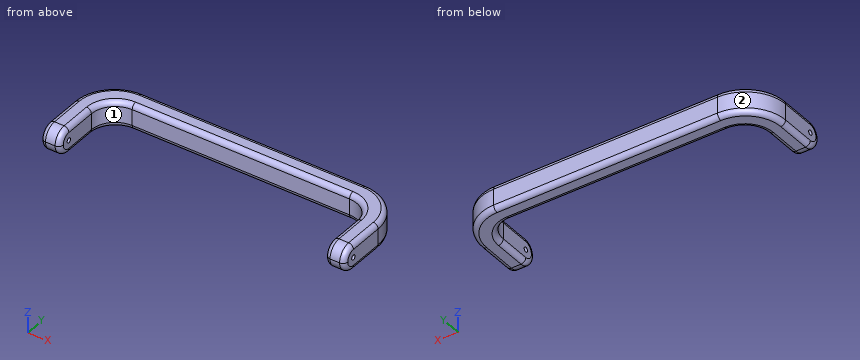
```python
from build123d import *

# Parameters (mm, degrees)
F1_DEPTH = 16
F2_R     = 15
F3_R     = 25
F4_R     = 7.99999
F5_R     = 1.5
F6_DEPTH = 250
F7_R     = 3


# Not quite as in the source:
# - a fillet or chamfer is up to 0.001 mm smaller than in the source, because OpenCascade refuses the exact size


with BuildPart() as f1:
    # F0 (on Top) → F1 (new body)
    with BuildSketch(Plane.XY):
        Polygon((95, 35.7796452148), (0, 35.7796452148), (-95, 35.7796452148), (-95, -19.2203547852), (-83, -19.2203547852), (-83, 23.7796452148), (0, 23.7796452148), (83, 23.7796452148), (83, -19.2203547852), (95, -19.2203547852), align=None)
    extrude(amount=F1_DEPTH)

    # F2
    f2_edges = [f1.edges().sort_by_distance(p)[0] for p in [
        (-83, 23.779645, 8),
        (83, 23.779645, 8),
    ]]
    fillet(f2_edges, radius=F2_R)

    # F3
    f3_edges = [f1.edges().sort_by_distance(p)[0] for p in [
        (-95, 35.779645, 8),
        (95, 35.779645, 8),
    ]]
    fillet(f3_edges, radius=F3_R)

    # F4 (radius 8 in the source; OpenCascade refuses exactly that, so slightly less here)
    f4_edges = [f1.edges().sort_by_distance(p)[0] for p in [
        (-89, -19.220355, 16),
        (-89, -19.220355, 0),
        (89, -19.220355, 16),
        (89, -19.220355, 0),
    ]]
    fillet(f4_edges, radius=F4_R)

    # F5 (on face) → F6 (cut)
    with BuildSketch(Plane.YZ.offset(95)):
        with Locations((-11.2203547852, 8)):
            Circle(F5_R)
    extrude(amount=-F6_DEPTH, mode=Mode.SUBTRACT)

    # F7
    f7_edges = [f1.edges().sort_by_distance(p)[0] for p in [
        (-95, -0.22036, 0),
        (-89, -11.220365, 0),
        (-87.67767, 28.457315, 0),
        (-83, -1.22036, 0),
        (0, 35.779645, 0),
        (-78.606602, 19.386247, 0),
        (87.67767, 28.457315, 0),
        (0, 23.779645, 0),
        (95, -0.22036, 0),
        (78.606602, 19.386247, 0),
        (89, -11.220365, 0),
        (83, -1.22036, 0),
    ]]
    fillet(f7_edges, radius=F7_R)


solid = f1.part
```
The listing builds one solid part. Answer for the finished solid, in the listing's coordinates (mm). Face numbers are marked on the shaded views. Coordinates: 2 decimals unless noted, no trailing zeros. Loops run counter-clockwise (first coordinate to the right, second up) from the corner with the lowest first, then second, coordinate; pieces in that order, holes last. Notation, with made-up numbers: (73.25, 61.25) - (77.25, 61.25) arc R11 cw to (77.25, 67.25) - close; hole circle Ø9 at (-3.5, 34.5). An arc over 180 degrees is marked (long way). Use a Markdown table: item, result. Add a question column.
1) The part is cut by section A-A, the plane x = -42. Give the vertices of the cut face in (y, z).
2) Given pin 1 (4 mm diameter, centred on x = -65, z = 9, fed in from -Y); pin 2 (1 mm diameter, centred on y = 21, z = 7, fed in from -X); pin 3 (4 mm diameter, centred on y = 29, z = 12, fed in from -X), each flat-ended and moving along its own axis, determine where each tip first touches the part or whether it passes through.
3) Find the intervals of material crossed by line 1 (X direction, y = -10.5, z = 4.5); line 2 (Y direction, x = 62, z = 9.25); line 3 (X direction, y = 3, z = 1.5), in increasing order.
4) The mould has two halves that part along Y. Classify the marked faces 1 and 2: released by +Y, released by -Y, zero draft, split by the parting line, or undercut.
Here are the results:
| question | item | result |
|---|---|---|
| 1 | outline | (23.78, 3) arc R3 ccw to (26.78, 0) - (32.78, 0) arc R3 ccw to (35.78, 3) - (35.78, 13) arc R3 ccw to (32.78, 16) - (26.78, 16) arc R3 ccw to (23.78, 13) - close |
| 2 | pin 1 | stops at y = 23.78 |
| 2 | pin 2 | stops at x = -93.03 |
| 2 | pin 3 | stops at x = -89.02 |
| 3 | line 1 | x = -95 to -83, 83 to 95 |
| 3 | line 2 | y = 23.78 to 35.78 |
| 3 | line 3 | x = -94.6 to -83.4, 83.4 to 94.6 |
| 4 | face 1 | released by -Y |
| 4 | face 2 | released by +Y |
